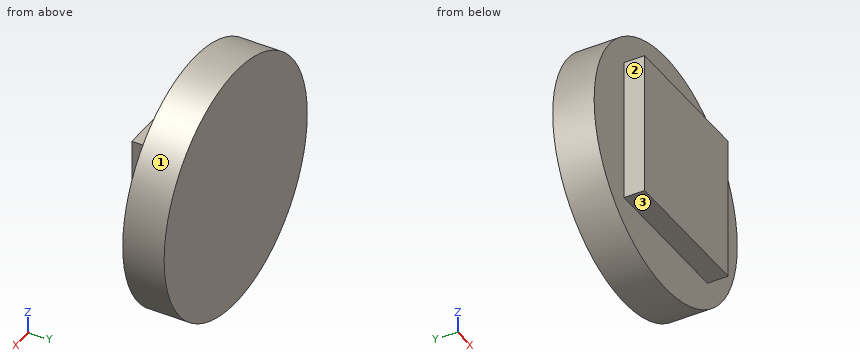
Autodesk Inventor part; units mm, degrees
ref_plane "YZ Plane" through (0, 0, 0) normal (1, 0, 0) x (0, 1, 0)
ref_plane "XZ Plane" through (0, 0, 0) normal (0, 1, 0) x (-1, 0, 0)
ref_plane "XY Plane" through (0, 0, 0) normal (0, 0, 1) x (1, 0, 0)
sketch "草图1" plane through (0, 0, 0) normal (0, 1, 0) x (-1, 0, 0)
  circle A0 centre (0, 0) radius 30
  dimension "d0" = 60
extrude "拉伸1" add sketch "草图1" along normal blind 10
sketch "草图2" plane through (0, 0, 0) normal (0, -1, 0) x (1, 0, 0)
  line L0 (-17.5, -17.5) -> (17.5, -17.5)
  line L1 (17.5, -17.5) -> (17.5, 17.5)
  line L2 (17.5, 17.5) -> (-17.5, 17.5)
  line L3 (-17.5, 17.5) -> (-17.5, -17.5)
  line L4 (-17.5, -17.5) -> (17.5, 17.5) construction
  line L5 (17.5, -17.5) -> (-17.5, 17.5) construction
  point P0 (0, 0)
  dimension "d3" = 35
  dimension "d4" = 35
extrude "拉伸2" add sketch "草图2" along normal blind 5
properties part number "底座"
For this review, take the finished solid that the model builds, in its own axes (mm). Face numbers are marked on the shaded views. A direction names the side the tool comes from. Coordinates: 2 decimals unless noted, no trailing zeros. Loops run counter-clockwise (first coordinate to the right, second up) from the corner with the lowest first, then second, coordinate; pieces in that order, holes last. Notation, with made-up numbers: (81, 40) -> (96, 40) arc R27 cw to (96, 66) -> close; hole circle Ø3 at (-25, 71). An arc over 180 degrees is marked (long way). Return JSON: item names as keys, results as strings. Group by question number.
(1) To check wall thickness, follow L1, parallel to Z at x = -13, y = -3; L2, parallel to Y at x = -19, z = -14; L3, parallel to X at y = 2.5, z = -1. State the ranges of each line that lie inside material, in increasing order.
(2) For pin 1 Ø5.5 at (y, z) = (-3.5, 4) entering from +X; pin 2 Ø3 at (y, z) = (6, 18.5) entering from -X; pin 3 Ø4 at (y, z) = (-1.5, 7) entering from -X, all flat-tipped, find the tip position at first contact; note any pin that passes through.
(3) Consider section D-D, the plane y = 8.75. Give the boundary of the cut face in (x, z), plus the area to 3 significant figures.
(4) Consider section A-A, the plane x = 0. Give the boundary of the cut face in (y, z), plus the area to 3 significant figures.
(5) Tool access review of the marked faces 1, 2 and 3: name each direction out of +Z, -Z, +X, -X, +Y, -Y from which nothing blocks a thin tool from reaching the whole face with its end or side.
(6) Consider section B-B, the plane z = 0. Give the boundary of the cut face in (x, y).
(7) Consider section C-C, the plane y = -4. Give the boundary of the cut face in (x, z), plus the area to 4 significant figures.
Results below:
{
 "1": {"L1": "z = -17.5 to 17.5", "L2": "y = 0 to 10", "L3": "x = -29.98 to 29.98"},
 "2": {"pin 1": "stops at x = 17.5", "pin 2": "stops at x = -24.72", "pin 3": "stops at x = -29.46"},
 "3": {"outline": "circle Ø60 at (0, 0)", "area": "2,830 mm2"},
 "4": {"outline": "(-5, -17.5) -> (0, -17.5) -> (0, -30) -> (10, -30) -> (10, 30) -> (0, 30) -> (0, 17.5) -> (-5, 17.5) -> close", "area": "775 mm2"},
 "5": {"face 1": "+Y, -Y", "face 2": "+Z, -Z, -X, -Y", "face 3": "-Z, +X, -X, -Y"},
 "6": {"outline": "(-30, 0) -> (-17.5, 0) -> (-17.5, -5) -> (17.5, -5) -> (17.5, 0) -> (30, 0) -> (30, 10) -> (-30, 10) -> close"},
 "7": {"outline": "(-17.5, -17.5) -> (17.5, -17.5) -> (17.5, 17.5) -> (-17.5, 17.5) -> close", "area": "1,225 mm2"}
}
